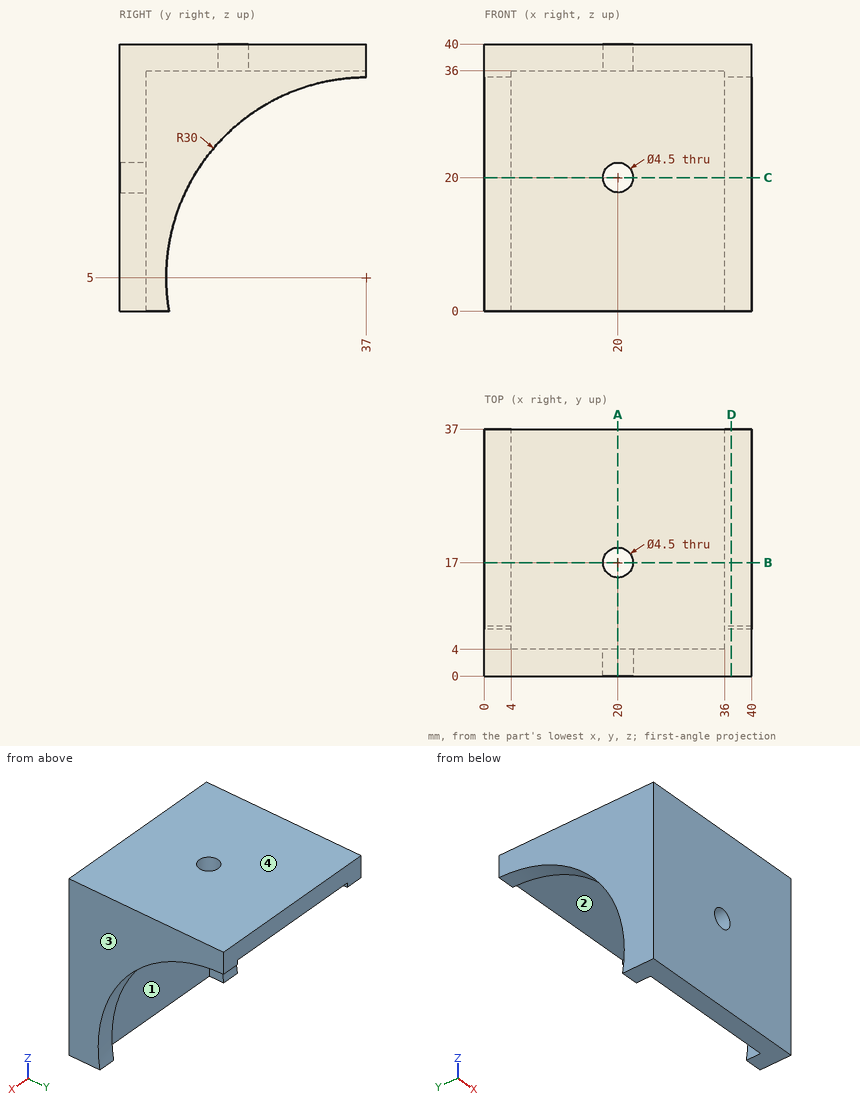
Design review of the part shown in the three views and the two pictorial views. Dimensions are in mm from the part's minimum x, y and z. Give positions to 0.01 mm unless a question says otherwise; leave off trailing zeros. Loops run counter-clockwise (first coordinate to the right, second up) from the corner with the lowest first, then second, coordinate; pieces in that order, holes last. Notation, with made-up numbers: (45.25, -8.5) -> (99.25, -8.5) arc R36 cw to (99.25, 27.5) -> close; hole circle Ø11 at (30, -6.5). An arc over 180 degrees is marked (long way). Answer as a JSON object with one key per item and string values. Group by question number.
Q1. Insertion check: pin 1 (9.5 mm diameter, centred on x = 25, y = 26.5, fed in from -Z); pin 2 (7 mm diameter, centred on x = 20, z = 20, fed in from +Y). Each pin has a flat end and moves straight along its axis. Give the tip position at first contact, or say it passes through.
Q2. Take a section at B-B (y = 17). Write out the cut boundary in (x, z).
Q3. Wall thickness on line 1 along X through (y, z) = (17, 39); line 2 along Y through (x, z) = (20, 38.8); line 3 along X through (y, z) = (10, 21): over which ranges is each line inside the solid? List them lowest first.
Q4. Take a section at D-D (x = 37). Write out the cut boundary in (y, z), plus the area to 3 significant figures.
Q5. Take a section at C-C (z = 20). Write out the cut boundary in (x, y).
Q6. Take a section at A-A (x = 20). Write out the cut boundary in (y, z), plus the area to 3 significant figures.
Q7. Draft analysis for pull direction X (two halves, no side actions). For the marked faces 1, 2, 3 and 4, state which applies: pulls with the +X half, pulls with the -X half, needs draft (parallel to the pull), parting line crosses it, or undercut.
Answer below:
{
 "1": {"pin 1": "stops at z = 36", "pin 2": "stops at y = 4"},
 "2": {"outline": "(0, 27.36) -> (4, 27.36) -> (4, 36) -> (17.75, 36) -> (17.75, 40) -> (0, 40) -> close; (22.25, 36) -> (36, 36) -> (36, 27.36) -> (40, 27.36) -> (40, 40) -> (22.25, 40) -> close"},
 "3": {"line 1": "x = 0 to 17.75, 22.25 to 40", "line 2": "y = 0 to 14.75, 19.25 to 37", "line 3": "x = 0 to 4, 36 to 40"},
 "4": {"outline": "(0, 0) -> (7.42, 0) arc R30 cw to (37, 35) -> (37, 40) -> (0, 40) -> close", "area": "624 mm2"},
 "5": {"outline": "(0, 0) -> (17.75, 0) -> (17.75, 4) -> (4, 4) -> (4, 11.02) -> (0, 11.02) -> close; (22.25, 0) -> (40, 0) -> (40, 11.02) -> (36, 11.02) -> (36, 4) -> (22.25, 4) -> close"},
 "6": {"outline": "(0, 0) -> (4, 0) -> (4, 17.75) -> (0, 17.75) -> close; (0, 22.25) -> (4, 22.25) -> (4, 36) -> (14.75, 36) -> (14.75, 40) -> (0, 40) -> close; (19.25, 36) -> (37, 36) -> (37, 40) -> (19.25, 40) -> close", "area": "256 mm2"},
 "7": {"face 1": "undercut", "face 2": "undercut", "face 3": "pulls with the +X half", "face 4": "needs draft"}
}
